```python
from build123d import *

# Parameters (mm, degrees)
SKETCH001_R     = 1.7
POCKET_DEPTH    = 5.001
SKETCH002_R     = 2.95
POCKET001_DEPTH = 3
SKETCH003_W     = 10
SKETCH003_H     = 1
POCKET002_DEPTH = 10


with BuildPart() as part:
    # Sketch → Revolution (revolve)
    with BuildSketch(Plane.XZ):
        Polygon((30.2, 0), (30.2, 15), (29.2, 15), (29.2, 5), (21, 5), (21, 0), align=None)
    revolve(axis=Axis((0, 0, 0), (0, 0, 1)))

    # Sketch001 (on Face4 of Revolution) → Pocket (cut, through all)
    with BuildSketch(Plane(origin=(0, 0, 5), x_dir=(-1, 0, 0), z_dir=(0, 0, 1))):
        with Locations((24, 0)):
            Circle(SKETCH001_R)
        with Locations((0, 24)):
            Circle(SKETCH001_R)
        with Locations((-24, 0)):
            Circle(SKETCH001_R)
        with Locations((0, -24)):
            Circle(SKETCH001_R)
    extrude(amount=-POCKET_DEPTH, mode=Mode.SUBTRACT)

    # Sketch002 (on Face10 of Pocket) → Pocket001 (cut)
    with BuildSketch(Plane(origin=(0, 0, 5), x_dir=(-1, 0, 0), z_dir=(0, 0, 1))):
        with Locations((0, 24)):
            Circle(SKETCH002_R)
        with Locations((-24, 0)):
            Circle(SKETCH002_R)
        with Locations((0, -24)):
            Circle(SKETCH002_R)
        with Locations((24, 0)):
            Circle(SKETCH002_R)
    extrude(amount=-POCKET001_DEPTH, mode=Mode.SUBTRACT)

    # Sketch003 (on Face3 of Pocket001) → Pocket002 (cut)
    with BuildSketch(Plane(origin=(0, 0, 15), x_dir=(-1, 0, 0), z_dir=(0, 0, 1))):
        with Locations((-30, 0)):
            Rectangle(SKETCH003_W, SKETCH003_H)
    extrude(amount=-POCKET002_DEPTH, mode=Mode.SUBTRACT)


solid = part.part
```
Check sheet for the modelled part. Datum: model origin and axes. Units: mm. A direction names the side the tool comes from. Give positions to 0.01 mm unless a question says otherwise; leave off trailing zeros. Order: outer loops, then holes, each group sorted by start corner. A loop starts at its lowest first (then second) coordinate and runs counter-clockwise, first axis right, second up. Notation, with made-up numbers: M 81.5,-25 L 113.5,-25 A9 cw 113.5,-15 Z; hole C 35,86.25 d7. An arc over 180 degrees is marked long. Answer in a Markdown table with one row per item. Add a question column.
Q1. Sectioned sample at C-C, the plane z = 6. Record the boundary of the cut face in (x, y), and give its area (3 significant figures).
Q2. Thickness scan on L1, parallel to Y at x = 26.5, z = 4; L2, parallel to Y at x = 6, z = 1.75; L3, parallel to Z at x = 26, y = -4.5. Record the ranges inside material, lowest first.
Q3. Release check for a two-part mould opening along Y. For faces 3 (the flat face through (0, -22, 2)), 4 (the flat face through (-25, 16, 15)), 5 (the cylindrical face through (-6.55, -29.48, 7.6)) record: released by +Y, released by -Y, zero draft, split by the parting line, or undercut.
Q4. Sectioned sample at B-B, the plane x = 20. Record the boundary of the cut face in (y, z).
Q5. Gauge pin test, flat ends, axial feed: pin 1 Ø1.5 at (x, z) = (1.5, 8.5) entering from -Y; pin 2 Ø2 at (x, y) = (0, -24) entering from +Z; pin 3 Ø2 at (y, z) = (-19.5, 7.5) entering from +X; pin 4 Ø1.8 at (x, y) = (25, -1.5) entering from +Z. Record the tip position at first contact, or that the pin passes through.
Q6. Sectioned sample at A-A, the plane y = 19. Record the boundary of the cut face in (x, z).
Q7. Sectioned sample at D-D, the plane x = -24. Record the boundary of the cut face in (y, z).
Q8. Access from +Z, -Z, +X, -X, +Y, -Y to the whole of each face (thin tool, end or side, straight path). Record for faces 1 (the cylindrical face through (-29.17, 1.28, 9.93)), 2 (the cylindrical face through (-25.57, 0.65, 1.01)).
Verdict:
| question | item | result |
|---|---|---|
| 1 | outline | M 29.2,-0.5 A29.2 cw long 29.2,0.5 L 30.2,0.5 A30.2 ccw long 30.2,-0.5 Z |
| 1 | area | 186 mm² |
| 2 | L1 | -14.48 to -1.57, 1.57 to 14.48 |
| 2 | L2 | -29.6 to -20.12, 20.12 to 29.6 |
| 2 | L3 | 0 to 5 |
| 3 | face 3 | undercut |
| 3 | face 4 | zero draft |
| 3 | face 5 | split by the parting line |
| 4 | outline | M -22.63,0 L -6.4,0 L -6.4,5 L -21.28,5 L -21.28,15 L -22.63,15 Z; M 6.4,0 L 22.63,0 L 22.63,15 L 21.28,15 L 21.28,5 L 6.4,5 Z |
| 5 | pin 1 | y = -30.19 |
| 5 | pin 2 | through |
| 5 | pin 3 | x = 23.87 |
| 5 | pin 4 | z = 2 |
| 6 | outline | M -23.47,0 L -8.94,0 L -8.94,5 L -22.17,5 L -22.17,15 L -23.47,15 Z; M 8.94,0 L 23.47,0 L 23.47,15 L 22.17,15 L 22.17,5 L 8.94,5 Z |
| 7 | outline | M -18.33,0 L -1.7,0 L -1.7,2 L -2.95,2 L -2.95,5 L -16.63,5 L -16.63,15 L -18.33,15 Z; M 1.7,0 L 18.33,0 L 18.33,15 L 16.63,15 L 16.63,5 L 2.95,5 L 2.95,2 L 1.7,2 Z |
| 8 | face 1 | +Z |
| 8 | face 2 | +Z, -Z |
